Source: CAD feature listing. Evaluate the final solid. Frame: model axes, mm. A direction names the side the tool comes from. Round coordinates to 2 decimals unless told otherwise and drop trailing zeros. Order: outer loops, then holes, each group sorted by start corner. A loop starts at its lowest first (then second) coordinate and runs counter-clockwise, first axis right, second up.
Autodesk Inventor part; units mm, degrees
ref_plane "YZ Plane" through (0, 0, 0) normal (1, 0, 0) x (0, 1, 0)
ref_plane "XZ Plane" through (0, 0, 0) normal (0, 1, 0) x (-1, 0, 0)
ref_plane "XY Plane" through (0, 0, 0) normal (0, 0, 1) x (1, 0, 0)
sketch "Sketch1" plane through (0, 0, 0) normal (0, 0, 1) x (1, 0, 0)
  line L0 (11.75, -37) -> (22.75, -37)
  line L1 (11.75, -37) -> (0.75, -37)
  line L2 (0.75, -37) -> (0.75, -32)
  line L3 (0.75, -32) -> (22.75, -32)
  line L4 (22.75, -32) -> (22.75, -37)
  line L5 (0.75, -32) -> (0.75, 6.35)
  line L6 (22.75, -32) -> (47, -32)
  line L7 (47, -32) -> (47, 6.35)
  line L8 (0.75, 6.35) -> (0.75, 9.525)
  line L9 (0.75, 9.525) -> (47, 9.525)
  line L10 (47, 9.525) -> (47, 6.35)
  point P0 (0, 0)
  dimension "d2" = 11
  dimension "d3" = 11
  dimension "d4" = 5
extrude "Extrusion1" add sketch "Sketch1" along normal mid plane 26 contours L3 L5 L8 L9 L10 L7 L6
sketch "Sketch2" plane through (0.75, 9.525, 13) normal (0, 1, 0) x (1, 0, 0)
  line L0 (0, 26) -> (0, 0)
  line L1 (0, 13) -> (11, 13)
  circle A0 centre (11, 13) radius 10.5
  point P0 (-0.75, 13)
  dimension "d7" = 11
  dimension "d8" = 21
extrude "Extrusion2" cut sketch "Sketch2" against normal blind 1
sketch "Sketch3" plane through (0.75, -32, 13) normal (0, -1, 0) x (1, 0, 0)
  line L0 (0, -26) -> (0, 0)
  line L1 (46.25, -26) -> (46.25, 0)
  line L2 (0, -13) -> (11, -13)
  circle A0 centre (11, -13) radius 11
  point P0 (-0.75, -13)
  dimension "d11" = 11
  dimension "d12" = 22
extrude "Extrusion3" add sketch "Sketch3" along normal blind 5
fillet "Fillet1" radius 2 11 edges at (47, -11.2375, 13) (47, -32, 0) (47, -11.2375, -13) (47, 9.525, 0) (23.875, 9.525, 13) (23.875, -32, 13) (23.875, -32, -13) (0.75, -11.2375, 13) (0.75, 9.525, 0) (0.75, -11.2375, -13) (23.875, 9.525, -13)
properties part number "Wrist2"
1. Section D-D on z = 2.75. Return loops of the section in (x, y) (3 decimals).
2. First-contact query: pin 1 (6 mm diameter, centred on x = 30.5, z = -9, fed in from -Y); pin 2 (6.5 mm diameter, centred on x = 11.5, z = -0.5, fed in from +Y) (3 decimals). Flat tips, straight axial feed; report the tip coordinate or a pass-through.
3. Line query: line 1 along Y through (x, z) = (14.5, -7.75) (3 decimals); line 2 along Y through (x, z) = (23, -0.5) (3 decimals); line 3 along Z through (x, y) = (11.75, 9.25). Output: solid intervals per line, ascending.
4. Section C-C on x = 9. Return loops of the section in (y, z) (3 decimals), plus the area to 3 significant figures.
5. Access query for faces 1 (the face through (3, -32, 8)), 2 (the face through (21.765, 9.032, -3.154)), 3 (the face through (9.37, -34.47, 10.74)), 4 (the face through (3, -32, -8)). Directions: +Z, -Z, +X, -X, +Y, -Y. A direction counts if a zero-diameter tool reaches every point of the face in a straight line with its end or side. Return the directions, or none.
6. Section A-A on x = 31. Return loops of the section in (y, z) (3 decimals), plus the area to 3 significant figures.
7. Section B-B on z = 9.5. Return loops of the section in (x, y) (3 decimals), plus the area to 3 significant figures.
Result:
1. outline: (0.75, -32) - (1.099, -32) - (1.099, -37) - (22.401, -37) - (22.401, -32) - (45, -32) arc R2 ccw to (47, -30) - (47, 7.525) arc R2 ccw to (45, 9.525) - (21.883, 9.525) - (21.883, 8.525) - (1.617, 8.525) - (1.617, 9.173) arc R2 ccw to (0.75, 7.525) - close
2. pin 1: stops at y = -32
2. pin 2: stops at y = 8.525
3. line 1: y = -37 to 8.525
3. line 2: y = -32 to 9.525
3. line 3: z = -12.01 to -10.5, 10.5 to 12.01
4. outline: (-37, -10.651) - (-32, -10.651) - (-32, -11) arc R2 ccw to (-30, -13) - (7.525, -13) arc R2 ccw to (9.525, -11) - (9.525, -10.133) - (8.525, -10.133) - (8.525, 10.133) - (9.525, 10.133) - (9.525, 11) arc R2 ccw to (7.525, 13) - (-30, 13) arc R2 ccw to (-32, 11) - (-32, 10.651) - (-37, 10.651) - close
4. area: 1,160 mm2
5. face 1: +Z, -X, -Y
5. face 2: +Y
5. face 3: -Y
5. face 4: -Z, -X, -Y
6. outline: (-32, -11) arc R2 ccw to (-30, -13) - (7.525, -13) arc R2 ccw to (9.525, -11) - (9.525, 11) arc R2 ccw to (7.525, 13) - (-30, 13) arc R2 ccw to (-32, 11) - close
6. area: 1,080 mm2
7. outline: (0.75, -32) - (6.205, -32) - (6.205, -37) - (17.295, -37) - (17.295, -32) - (45, -32) arc R2 ccw to (47, -30) - (47, 7.525) arc R2 ccw to (45, 9.525) - (16.222, 9.525) - (16.222, 8.525) - (7.278, 8.525) - (7.278, 9.525) - (2.75, 9.525) arc R2 ccw to (0.75, 7.525) - close
7. area: 1,960 mm2
